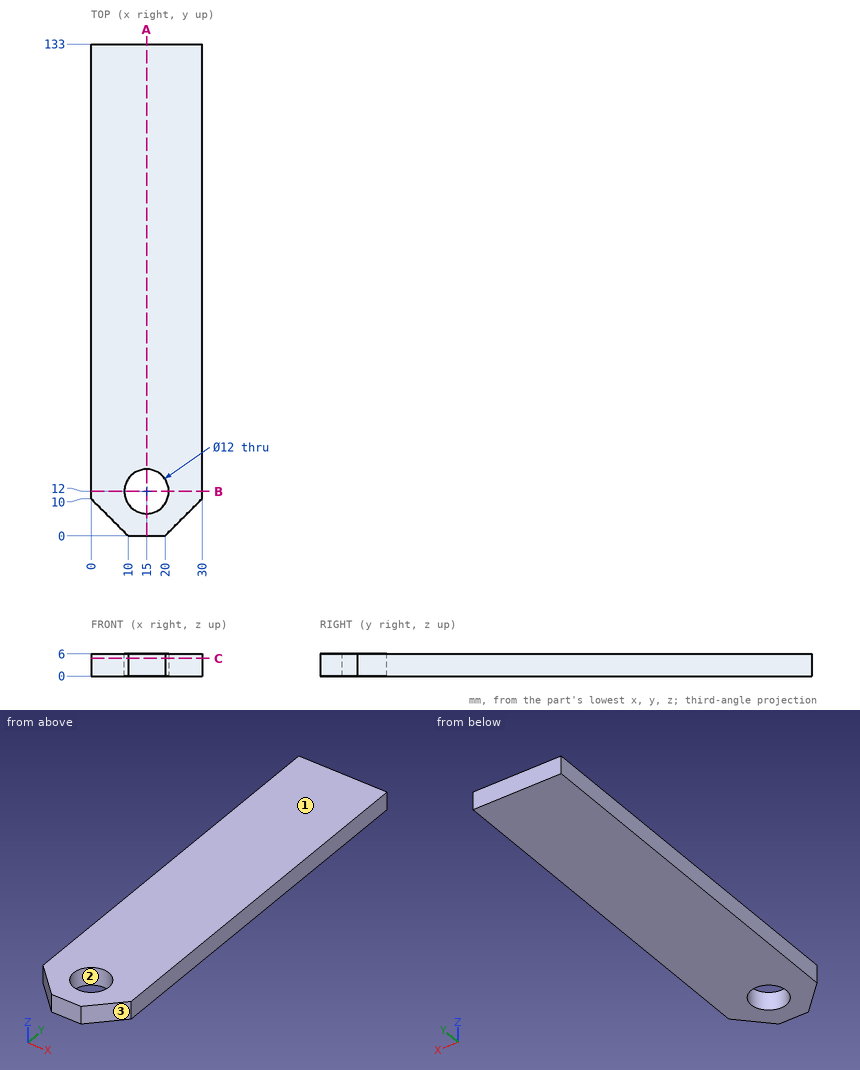
Design review of the part shown in the three views and the two pictorial views. Dimensions are in mm from the part's minimum x, y and z. Coordinates: 2 decimals unless noted, no trailing zeros. Loops run counter-clockwise (first coordinate to the right, second up) from the corner with the lowest first, then second, coordinate; pieces in that order, holes last. Notation, with made-up numbers: M 14,50.25 L 35,50.25 A15 cw 35,70.25 Z; hole C 79.25,56 d3. An arc over 180 degrees is marked long. Put each result on its own line as item: value. Start each with the question number.
Q1. Add section C-C (z = 4.75). Write out the cut boundary in (x, y), and give its area (3 significant figures).
Q2. Wall thickness on line 1 (Y direction, x = 15, z = 2.3); line 2 (Y direction, x = 16.25, z = 0.6); line 3 (Y direction, x = 4, z = 2.85): over which ranges is each line inside the solid? List them lowest first.
Q3. Add section B-B (y = 12). Write out the cut boundary in (x, z), and give its area (3 significant figures).
Q4. Add section A-A (x = 15). Write out the cut boundary in (y, z).
Q5. The part is to be moulded in two halves that separate along X. For the marked faces 1, 2 and 3, say which applies: +X half, -X half, draft (parallel to the pull), parting line (faces both ways), or undercut.
Answers:
1. outline: M 0,10 L 10,0 L 20,0 L 30,10 L 30,133 L 0,133 Z; hole C 15,12 d12
1. area: 3,780 mm^2
2. line 1: y = 0 to 6, 18 to 133
2. line 2: y = 0 to 6.13, 17.87 to 133
2. line 3: y = 6 to 133
3. outline: M 0,0 L 9,0 L 9,6 L 0,6 Z; M 21,0 L 30,0 L 30,6 L 21,6 Z
3. area: 108 mm^2
4. outline: M 0,0 L 6,0 L 6,6 L 0,6 Z; M 18,0 L 133,0 L 133,6 L 18,6 Z
5. face 1: draft
5. face 2: undercut
5. face 3: +X half
